Source: CAD feature listing. Evaluate the final solid. Frame: model axes, mm. Face numbers are marked on the shaded views. A direction names the side the tool comes from. Round coordinates to 2 decimals unless told otherwise and drop trailing zeros. Write each loop counter-clockwise with the first axis right and the second up, starting at its lowest first coordinate (ties: lowest second). Pieces come first, ordered by that corner, then holes.
Autodesk Inventor part; units mm, degrees
ref_plane "YZ Plane" through (0, 0, 0) normal (1, 0, 0) x (0, 1, 0)
ref_plane "XZ Plane" through (0, 0, 0) normal (0, 1, 0) x (-1, 0, 0)
ref_plane "XY Plane" through (0, 0, 0) normal (0, 0, 1) x (1, 0, 0)
sketch "Sketch1" plane through (0, 0, 0) normal (0, 0, 1) x (1, 0, 0)
  line L0 (0, 0) -> (0, 47.913)
  line L1 (0, 0) -> (52.4, 0)
  line L2 (52.4, 0) -> (52.4, 51.52)
  line L3 (52.4, 51.52) -> (0, 47.913)
  line L4 (3, 44) -> (9, 44)
  line L5 (9, 44) -> (9, 36)
  line L6 (9, 36) -> (3, 36)
  line L7 (3, 36) -> (3, 44)
  line L8 (3, 31) -> (9, 31)
  line L9 (9, 31) -> (9, 23)
  line L10 (9, 23) -> (3, 23)
  line L11 (3, 23) -> (3, 31)
  line L12 (3, 18) -> (9, 18)
  line L13 (9, 18) -> (9, 10)
  line L14 (9, 10) -> (3, 10)
  line L15 (3, 10) -> (3, 18)
  line L16 (26.2, 0) -> (26.2, 49.7165) construction
  line L17 (49.4, 44) -> (43.4, 44)
  line L18 (43.4, 44) -> (43.4, 36)
  line L19 (43.4, 36) -> (49.4, 36)
  line L20 (49.4, 36) -> (49.4, 44)
  line L21 (49.4, 31) -> (43.4, 31)
  line L22 (43.4, 31) -> (43.4, 23)
  line L23 (43.4, 23) -> (49.4, 23)
  line L24 (49.4, 23) -> (49.4, 31)
  line L25 (49.4, 18) -> (43.4, 18)
  line L26 (43.4, 18) -> (43.4, 10)
  line L27 (43.4, 10) -> (49.4, 10)
  line L28 (49.4, 10) -> (49.4, 18)
  line L29 (0, 0) -> (0, -15)
  line L30 (0, -15) -> (8, -15)
  line L31 (8, -15) -> (8, 0)
  line L32 (52.4, 0) -> (52.4, -15)
  line L33 (52.4, -15) -> (44.4, -15)
  line L34 (44.4, -15) -> (44.4, 0)
  line L35 (22.2, 0) -> (30.2, 0)
  line L36 (30.2, 0) -> (30.2, -15)
  line L37 (30.2, -15) -> (22.2, -15)
  line L38 (22.2, -15) -> (22.2, 0)
  point P0 (3, 14)
  point P1 (3, 27)
  point P2 (3, 40)
  point P3 (6, 10)
  point P4 (6, 23)
  point P5 (6, 18)
  point P6 (6, 36)
  point P7 (6, 31)
  dimension "d0" = 47.913
  dimension "d1" = 52.4
  dimension "d2" = 51.52
  dimension "d3" = 6
  dimension "d4" = 8
  dimension "d5" = 6
  dimension "d6" = 8
  dimension "d7" = 6
  dimension "d8" = 8
  dimension "d9" = 3
  dimension "d10" = 3
  dimension "d11" = 3
  dimension "d12" = 10
  dimension "d13" = 5
  dimension "d14" = 5
  dimension "d17" = 15
  dimension "d18" = 8
  dimension "d19" = 8
  dimension "d20" = 15
  dimension "d21" = 8
  dimension "d22" = 15
  dimension "d24" = 14.2
extrude "Extrusion1" add sketch "Sketch1" along normal blind 6 contours L0 L3 L2 L1
extrude "Extrusion2" add sketch "Sketch1" along normal blind 6 contours L1 L31 L30 L29 | L1 L36 L37 L38 | L32 L33 L34 L1
properties part number "sort support V2 wall 1"
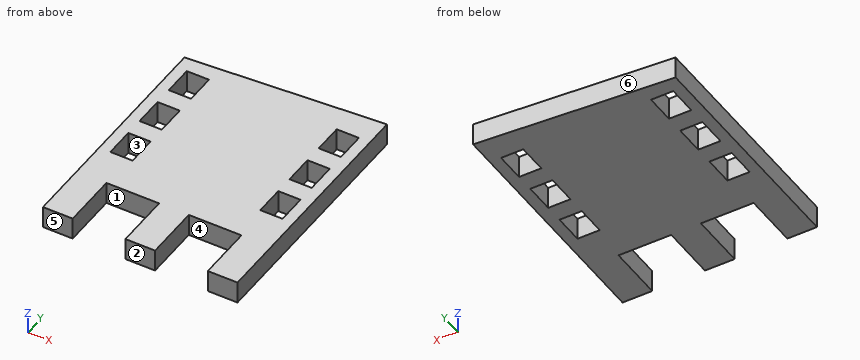
Q1. Section query B-B, the plane x = 47.5. Output: boundary loops of the cut face in (y, z).
Q2. Section query C-C, the plane z = 2. Give the number of separate pieces and of enclosed holes in the cut face, and give its area (3 significant figures).
Q3. Set-up query: the marked faces 1, 2 and 3. Return all of +Z, -Z, +X, -X, +Y, -Y with unobstructed straight access to the full face (end or side cutting, diameter ignored); none if empty.
Q4. Mould query, pull axis X, two halves, no side actions, for the marked faces 4, 5 and 6. Classes: pulls with the +X half, pulls with the -X half, needs draft (parallel to the pull), parting line crosses it, or undercut.
Q5. Line query: line 1 (X direction, y = -6, z = 0.35); line 2 (X direction, y = 27, z = 4.75); line 3 (Y direction, x = 48, z = 2.8). Output: solid intervals per line, ascending.
Q6. Section query A-A, the plane y = 14. Output: boundary loops of the cut face in (x, z), and give its area (3 significant figures).
Q7. Section query D-D, the plane x = 29. Output: boundary loops of the cut face in (y, z).
Q8. Pin query (flat end, axial travel): P1, Ø3, axis at x = 46, z = 2.5, coming from the +Y side; P2, Ø1, axis at x = 27.5, z = 4.5, coming from the +Y side; P3, Ø3, axis at x = 13, z = 1.5, coming from the +Y side. Return the tip coordinate at first contact, or that it passes through.
Filled in:
1. outline: (-15, 0) - (10, 0) - (10, 6) - (-15, 6) - close; (18, 0) - (23, 0) - (23, 6) - (18, 6) - close; (31, 0) - (36, 0) - (36, 6) - (31, 6) - close; (44, 0) - (51.18, 0) - (51.18, 6) - (44, 6) - close
2. separate pieces: 1
2. enclosed holes: 6
2. area: 2,680 mm2
3. face 1: +Z, -Z, -Y
3. face 2: +Z, -Z, +X, -X, -Y
3. face 3: +Z, -Z
4. face 4: undercut
4. face 5: needs draft
4. face 6: pulls with the -X half
5. line 1: x = 0 to 8, 22.2 to 30.2, 44.4 to 52.4
5. line 2: x = 0 to 3, 9 to 43.4, 49.4 to 52.4
5. line 3: y = -15 to 10, 18 to 23, 31 to 36, 44 to 51.22
6. outline: (0, 0) - (3, 0) - (3, 6) - (0, 6) - close; (9, 0) - (43.4, 0) - (43.4, 6) - (9, 6) - close; (49.4, 0) - (52.4, 0) - (52.4, 6) - (49.4, 6) - close
6. area: 242 mm2
7. outline: (-15, 0) - (49.91, 0) - (49.91, 6) - (-15, 6) - close
8. P1: stops at y = 51.18
8. P2: stops at y = 49.84
8. P3: stops at y = 48.91
